The listing builds one solid part. Answer for the finished solid, in the listing's coordinates (mm). Face numbers are marked on the shaded views. A direction names the side the tool comes from. Coordinates: 2 decimals unless noted, no trailing zeros. Loops run counter-clockwise (first coordinate to the right, second up) from the corner with the lowest first, then second, coordinate; pieces in that order, holes last. Notation, with made-up numbers: M 69.25,77 L 77.25,77 A22 ccw 77.25,105 Z; hole C 80,59.25 d11. An arc over 180 degrees is marked long. Answer as CSV lines item,"result". Start each with the question number.
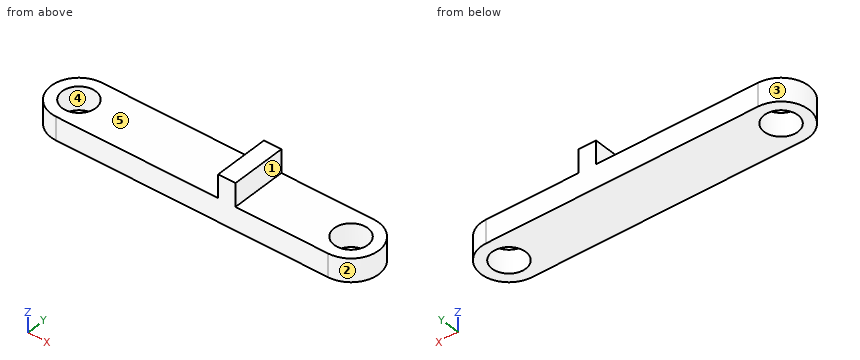
```python
from build123d import *

# Parameters (mm, degrees)
PAD_DEPTH    = 2
SKETCH001_R  = 1.45
POCKET_DEPTH = 2.001
SKETCH002_W  = 1.5
SKETCH002_H  = 4.8
PAD001_DEPTH = 2


with BuildPart() as part:
    # Sketch → Pad (new body)
    with BuildSketch(Plane.XY):
        with BuildLine():
            ThreePointArc((0, 2.4), (-2.4, 0), (0, -2.4))
            Line((0, -2.4), (23.5, -2.4))
            ThreePointArc((23.5, -2.4), (25.9, 0), (23.5, 2.4))
            Line((0, 2.4), (23.5, 2.4))
        make_face()
    extrude(amount=-PAD_DEPTH)

    # Sketch001 → Pocket (cut, through all)
    with BuildSketch(Plane.XY):
        Circle(SKETCH001_R)
        with Locations((23.5, 0)):
            Circle(SKETCH001_R)
    extrude(amount=-POCKET_DEPTH, mode=Mode.SUBTRACT)

    # Sketch002 → Pad001 (join)
    with BuildSketch(Plane.XY):
        with Locations((14.75, 0)):
            Rectangle(SKETCH002_W, SKETCH002_H)
    extrude(amount=PAD001_DEPTH)


solid = part.part
```
Item 1: Section A-A on y = 0 is taken. Determine the outline of the cut face in (x, z), then the cut area to 3 significant figures.
Item 2: For a pull along X with two mould halves and no side action, classify the marked faces 3, 4 and 5 as pulls with the +X half, pulls with the -X half, needs draft (parallel to the pull), parting line crosses it, or undercut.
Item 3: Each of these flat-tipped pins is pushed along its axis until it touches: P1, Ø2.5, axis at x = 5, y = 0, coming from the +Z side; P2, Ø2, axis at y = 0.5, z = 1.5, coming from the -X side. Where does it stop, or does it pass through?
Item 4: For the marked faces 1 and 2, determine the directions among +Z, -Z, +X, -X, +Y, -Y from which every point of the face is accessible in a straight line to the end or side of a thin tool.
Item 5: Section D-D on z = 0.75 is taken. Determine the outline of the cut face in (x, y).
Item 6: Consider line 1 (Y direction, x = 23.5, z = -0.4); line 2 (X direction, y = -0.3, z = -0.15); line 3 (X direction, y = 1.4, z = 0.95). Determine where each line is inside the solid, lowest interval first.
Item 7: Section B-B on z = -0.95 is taken. Determine the outline of the cut face in (x, y), then the cut area to 3 significant figures.
Item 8: Section C-C on y = 1.95 is taken. Determine the outline of the cut face in (x, z).
Results are:
1,outline,"M -2.4,-2 L -1.45,-2 L -1.45,0 L -2.4,0 Z; M 1.45,-2 L 22.05,-2 L 22.05,0 L 15.5,0 L 15.5,2 L 14,2 L 14,0 L 1.45,0 Z; M 24.95,-2 L 25.9,-2 L 25.9,0 L 24.95,0 Z"
1,area,"48.0 mm²"
2,face 3,"pulls with the -X half"
2,face 4,"undercut"
2,face 5,"needs draft"
3,P1,"z = 0"
3,P2,"x = 14"
4,face 1,"+Z, +X, +Y, -Y"
4,face 2,"+Z, -Z, +X"
5,outline,"M 14,-2.4 L 15.5,-2.4 L 15.5,2.4 L 14,2.4 Z"
6,line 1,"-2.4 to -1.45, 1.45 to 2.4"
6,line 2,"-2.38 to -1.42, 1.42 to 22.08, 24.92 to 25.88"
6,line 3,"14 to 15.5"
7,outline,"M 0,-2.4 L 23.5,-2.4 A2.4 ccw 23.5,2.4 L 0,2.4 A2.4 ccw Z; hole C 0,0 d2.9; hole C 23.5,0 d2.9"
7,area,"118 mm²"
8,outline,"M -1.4,-2 L 24.9,-2 L 24.9,0 L 15.5,0 L 15.5,2 L 14,2 L 14,0 L -1.4,0 Z"
